```python
from build123d import *

# Parameters (mm, degrees)
BOSS_EXTRUDE2_DEPTH = 0.254
CUT_EXTRUDE1_DEPTH  = 1.254
SKETCH13_W          = 444.5
SKETCH13_H          = 215.9
CUT_EXTRUDE3_DEPTH  = 1.254


with BuildPart() as part:
    # Sketch1 → Boss-Extrude2 (new body)
    with BuildSketch(Plane(origin=(0, 0, 0), x_dir=(0, 0, -1), z_dir=(1, 0, 0))):
        with BuildLine():
            Line((-222.25, 0), (-171.45, 0))
            Line((-171.45, 0), (-171.45, -215.9))
            ThreePointArc((-171.45, -215.9), (-165.870384182, -229.370384182), (-152.4, -234.95))
            Line((-152.4, -234.95), (152.4, -234.95))
            ThreePointArc((152.4, -234.95), (165.870384182, -229.370384182), (171.45, -215.9))
            Line((171.45, -215.9), (171.45, 0))
            Line((171.45, 0), (222.25, 0))
            Line((222.25, 0), (222.25, -266.7))
            ThreePointArc((222.25, -266.7), (216.670384182, -280.170384182), (203.2, -285.75))
            Line((203.2, -285.75), (-203.2, -285.75))
            ThreePointArc((-203.2, -285.75), (-216.670384182, -280.170384182), (-222.25, -266.7))
            Line((-222.25, -266.7), (-222.25, 0))
        make_face()
    extrude(amount=BOSS_EXTRUDE2_DEPTH)

    # Sketch11 → Cut-Extrude1 (cut, through all)
    with BuildSketch(Plane.ZY):
        with BuildLine():
            Line((-171.45, -103.759), (-180.975, -103.759))
            ThreePointArc((-180.975, -103.759), (-183.22006403, -104.68893597), (-184.15, -106.934))
            Line((-184.15, -106.934), (-184.15, -133.604))
            ThreePointArc((-184.15, -133.604), (-183.22006403, -135.84906403), (-180.975, -136.779))
            Line((-180.975, -136.779), (-171.45, -136.779))
            Line((-171.45, -136.779), (-171.45, -103.759))
        make_face()
        with BuildLine():
            Line((-44.45, -234.95), (-31.75, -234.95))
            Line((-31.75, -234.95), (-31.75, -244.475))
            ThreePointArc((-31.75, -244.475), (-32.67993597, -246.72006403), (-34.925, -247.65))
            Line((-34.925, -247.65), (-41.275, -247.65))
            ThreePointArc((-41.275, -247.65), (-43.52006403, -246.72006403), (-44.45, -244.475))
            Line((-44.45, -244.475), (-44.45, -234.95))
        make_face()
    cut_extrude1 = extrude(amount=-CUT_EXTRUDE1_DEPTH, mode=Mode.SUBTRACT)

    # Mirror2: Cut-Extrude1 across plane
    add(cut_extrude1.mirror(Plane.XY), mode=Mode.SUBTRACT)

    # Sketch13 → Cut-Extrude3 (cut, through all)
    with BuildSketch(Plane.ZY):
        with Locations((0, -107.95)):
            Rectangle(SKETCH13_W, SKETCH13_H)
    extrude(amount=-CUT_EXTRUDE3_DEPTH, mode=Mode.SUBTRACT)


solid = part.part
```
The listing builds one solid part. Answer for the finished solid, in the listing's coordinates (mm). Coordinates: 2 decimals unless noted, no trailing zeros. Loops run counter-clockwise (first coordinate to the right, second up) from the corner with the lowest first, then second, coordinate; pieces in that order, holes last. Notation, with made-up numbers: M 44,61.25 L 85,61.25 A8 cw 85,69.25 Z; hole C 72,-25 d5. An arc over 180 degrees is marked long. Answer as a JSON object with one key per item and string values. Group by question number.
Item 1: This flat-tipped pin is pushed along its axis until it touches: P1, Ø10, axis at y = -243.5, z = -9, coming from the -X side. Where does it stop, or does it pass through?
Item 2: Section B-B (y = -227) is taken. Write down the section's boundary in (x, z), and give its area (3 significant figures).
Item 3: Section D-D (z = 166) is taken. Write down the section's boundary in (x, y), and give its area (3 significant figures).
Item 4: Section C-C (z = 84) is taken. Write down the section's boundary in (x, y).
Item 5: Section A-A (x = 0.2) is taken. Write down the section's boundary in (y, z) (3 decimals), and give its area (3 significant figures).
Item 6: Consider L1, parallel to Y at x = 0.15, z = -10.5; L2, parallel to Z at x = 0.05, y = -230; L3, parallel to Z at x = 0.05, y = -233. Determine where each line is inside the solid, lowest interval first.
Solved:
{
 "1": {"P1": "stops at x = 0"},
 "2": {"outline": "M 0,-222.25 L 0.25,-222.25 L 0.25,-167.88 L 0,-167.88 Z; M 0,167.88 L 0.25,167.88 L 0.25,222.25 L 0,222.25 Z", "area": "27.6 mm2"},
 "3": {"outline": "M 0,-285.75 L 0.25,-285.75 L 0.25,-229.24 L 0,-229.24 Z", "area": "14.4 mm2"},
 "4": {"outline": "M 0,-285.75 L 0.25,-285.75 L 0.25,-234.95 L 0,-234.95 Z"},
 "5": {"outline": "M -285.75,-203.2 A19.05 ccw -266.7,-222.25 L -215.9,-222.25 L -215.9,-171.45 A19.05 cw -234.95,-152.4 L -234.95,-44.45 L -244.475,-44.45 A3.175 cw -247.65,-41.275 L -247.65,-34.925 A3.175 cw -244.475,-31.75 L -234.95,-31.75 L -234.95,31.75 L -244.475,31.75 A3.175 cw -247.65,34.925 L -247.65,41.275 A3.175 cw -244.475,44.45 L -234.95,44.45 L -234.95,152.4 A19.05 cw -215.9,171.45 L -215.9,222.25 L -266.7,222.25 A19.05 ccw -285.75,203.2 Z", "area": "24,200 mm2"},
 "6": {"L1": "y = -285.75 to -234.95", "L2": "z = -222.25 to -165.21, 165.21 to 222.25", "L3": "z = -222.25 to -160.8, 160.8 to 222.25"}
}
